Geometry check sheet. Reference: drawing and pictorial views, mm from the part's lowest x, y, z. A direction names the side the tool comes from. Give positions to 0.01 mm unless a question says otherwise; leave off trailing zeros. Order: outer loops, then holes, each group sorted by start corner. A loop starts at its lowest first (then second) coordinate and runs counter-clockwise, first axis right, second up.
Item 1: Sectioned sample at A-A on x = 12. Record the boundary of the cut face in (y, z), and give its area (3 significant figures).
Item 2: Access from +Z, -Z, +X, -X, +Y, -Y to the whole of each face (thin tool, end or side, straight path). Record for the marked faces 1, 2 and 3.
Item 3: Sectioned sample at B-B on z = 53.5. Record the boundary of the cut face in (x, y), and give its area (3 significant figures).
Item 4: Material ranges on line 1 along Y through (x, z) = (1.75, 46.5); line 2 along X through (y, z) = (246, 32), recorded low to high.
Item 5: Gauge pin test, flat ends, axial feed: P1, Ø5, axis at x = 11, y = 18, coming from the -Z side; P2, Ø7.5, axis at y = 249, z = 20, coming from the +X side; P3, Ø12.5, axis at y = 14.5, z = 41, coming from the -X side. Record the tip position at first contact, or that the pin passes through.
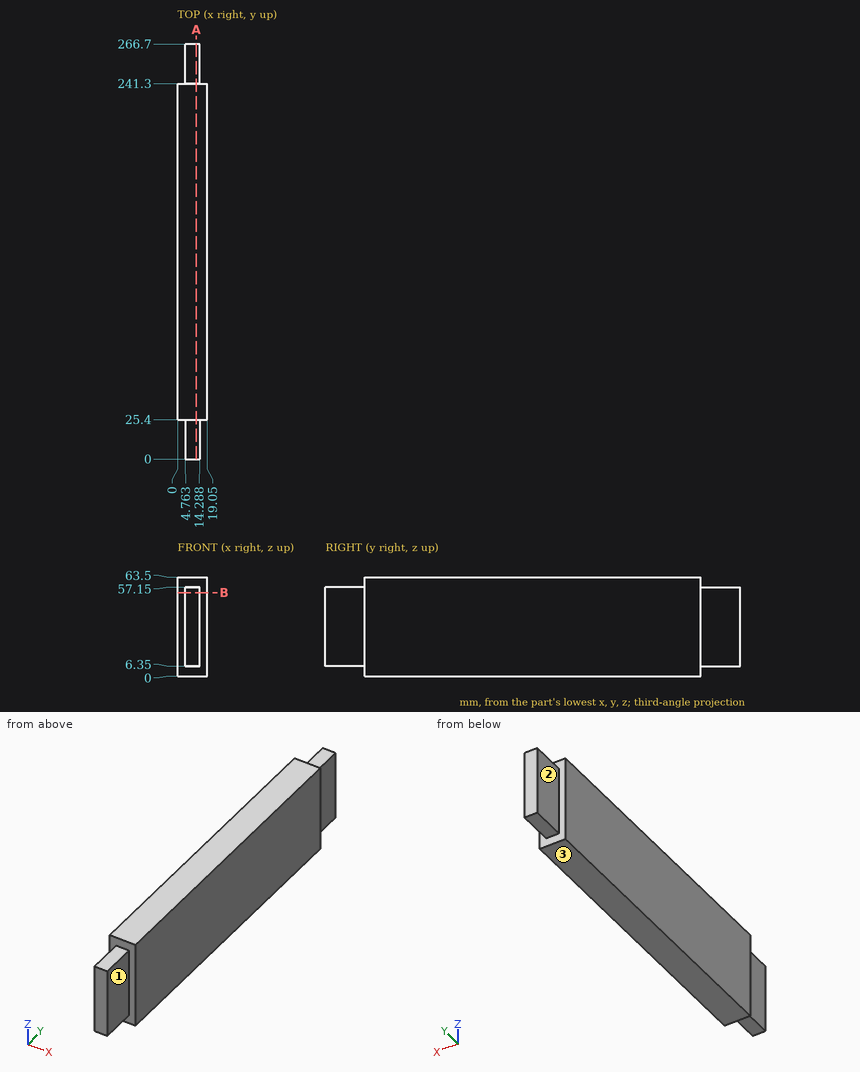
Report:
1. outline: (0, 6.35) - (25.4, 6.35) - (25.4, 0) - (241.3, 0) - (241.3, 6.35) - (266.7, 6.35) - (266.7, 57.15) - (241.3, 57.15) - (241.3, 63.5) - (25.4, 63.5) - (25.4, 57.15) - (0, 57.15) - close
1. area: 16,300 mm2
2. face 1: +Z, -Z, +X, -Y
2. face 2: +Z, -Z, -X, +Y
2. face 3: -Z, +X, -X, +Y, -Y
3. outline: (0, 25.4) - (4.76, 25.4) - (4.76, 0) - (14.29, 0) - (14.29, 25.4) - (19.05, 25.4) - (19.05, 241.3) - (14.29, 241.3) - (14.29, 266.7) - (4.76, 266.7) - (4.76, 241.3) - (0, 241.3) - close
3. area: 4,600 mm2
4. line 1: y = 25.4 to 241.3
4. line 2: x = 4.76 to 14.29
5. P1: stops at z = 6.35
5. P2: stops at x = 14.29
5. P3: stops at x = 4.76
